Check sheet for the modelled part. Datum: model origin and axes. Units: mm. A direction names the side the tool comes from. Give positions to 0.01 mm unless a question says otherwise; leave off trailing zeros. Use one line per item in the form item = value.
from build123d import *

# Parameters (mm, degrees)
ESQUISSE1_R                               = 30
BOSS_EXTRU_1_DEPTH                        = 5
ESQUISSE6_R                               = 35
ESQUISSE6_R_2                             = 30
BOSS_EXTRU_6_DEPTH                        = 10
ESQUISSE7_R                               = 32.5
ESQUISSE7_R_2                             = 30
BOSS_EXTRU_8_DEPTH                        = 30
CONG_2_R                                  = 10
BOSS_EXTRU_9_DEPTH                        = 20
BOSS_EXTRU_10_DEPTH                       = 12
CHANFREIN1_SIZE                           = 6
CONG_3_R                                  = 5
ENL_V_MAT_EXTRU_1_REACH                   = 93.085
ENL_V_MAT_EXTRU_1_END_RADIUS              = 32.5
ESQUISSE10_R                              = 4.5
ESQUISSE11_R                              = 4.5
ESQUISSE11_R_2                            = 2.6
BOSS_EXTRU_11_DEPTH                       = 3
R_P_TITION_CIRCULAIRE1_COUNT              = 4
CHANFREIN1_OF_R_P_TITION_CIRCULAIRE1_SIZE = 6


# Some blends are built 0.0001 mm under size
with BuildPart() as part:
    # Esquisse1 → Boss.-Extru.1 (new body)
    with BuildSketch(Plane.XY):
        with BuildLine():
            Line((-10.847469364, 35.896830061), (-80, 15))
            Line((-80, 15), (-80, -15))
            Line((-80, -15), (-10.847469364, -35.896830061))
            ThreePointArc((-10.847469364, -35.896830061), (37.5, 0), (-10.847469364, 35.896830061))
        make_face()
        Circle(ESQUISSE1_R, mode=Mode.SUBTRACT)
    extrude(amount=BOSS_EXTRU_1_DEPTH)

    # Esquisse6 → Boss.-Extru.6 (add)
    with BuildSketch(Plane.XY.offset(5)):
        Circle(ESQUISSE6_R)
        Circle(ESQUISSE6_R_2, mode=Mode.SUBTRACT)
    extrude(amount=BOSS_EXTRU_6_DEPTH)

    # Esquisse7 → Boss.-Extru.8 (add)
    with BuildSketch(Plane.XY.offset(15)):
        Circle(ESQUISSE7_R)
        Circle(ESQUISSE7_R_2, mode=Mode.SUBTRACT)
    extrude(amount=BOSS_EXTRU_8_DEPTH)

    # Congé2
    # the kernel refuses this fillet: 10 mm, written as the material it adds along each edge
    with BuildSketch(Plane(origin=(0, 0, 15), x_dir=(1, 0, 0), z_dir=(0, -1, 0))) as cong_2_piece_1:
        with BuildLine():
            CenterArc((42.5, 6.614378278), CONG_2_R, 180, 41.409622109)
            Line((32.5, 6.614378278), (32.3, 6.614378278))
            Line((32.3, 6.614378278), (32.3, 0))
            Line((32.3, 0), (32.5, -0.2))
            ThreePointArc((32.5, -0.2), (33.75, -0.2), (34.85, -0.132287566))
            Line((34.85, -0.132287566), (35, 0))
        make_face()
    revolve(axis=Axis((0, 0, 15), (0, 0, 1)))

    # Esquisse8 → Boss.-Extru.9 (add)
    with BuildSketch(Plane.XY.offset(5)):
        with BuildLine():
            Line((-80, 15), (-37.080992435, 15))
            ThreePointArc((-37.080992435, 15), (-40, 0), (-37.080992435, -15))
            Line((-37.080992435, -15), (-80, -15))
            Line((-80, -15), (-80, 15))
        make_face()
    extrude(amount=BOSS_EXTRU_9_DEPTH)

    # Esquisse9 → Boss.-Extru.10 (add)
    with BuildSketch(Plane.XY.offset(45)):
        Polygon((-29.606282822, -13.405894878), (-22.723365586, -23.235719409), (-16.170149231, -18.647107918), (-23.053066468, -8.817283387), align=None)
    boss_extru_10 = extrude(amount=-BOSS_EXTRU_10_DEPTH)

    # Chanfrein1
    # the kernel refuses this chamfer: 6 mm, written as the material it adds along each edge
    with BuildSketch(Plane(origin=(0, 0, 33), x_dir=(-0.2418024484236128, -0.9703254999928355, 0), z_dir=(0.9703254999928355, -0.2418024484236128, 0))) as chanfrein1_piece_1_section:
        Polygon((30, CHANFREIN1_SIZE), (30 - CHANFREIN1_SIZE, 0), (30, 0), align=None)
    chanfrein1_piece_1 = revolve(axis=Axis((0, 0, 33), (0, 0, -1)), revolution_arc=82.01410645, mode=Mode.PRIVATE)
    chanfrein1_piece_1 = split(chanfrein1_piece_1, bisect_by=Plane(origin=(-19.354245876, -20.876636392, 31.008979001), z_dir=(-0.573576436351043, 0.819152044288994, 0)), keep=Keep.TOP, mode=Mode.PRIVATE)
    chanfrein1_piece_1 = split(chanfrein1_piece_1, bisect_by=Plane(origin=(-26.237163113, -11.04681186, 31.008979001), z_dir=(0.5735764363510415, -0.8191520442889951, 0)), keep=Keep.TOP, mode=Mode.PRIVATE)
    chanfrein1_piece_1 = split(chanfrein1_piece_1, bisect_by=Plane(origin=(-19.611607849, -13.732195653, 31.008979001), z_dir=(-0.8191520442889946, -0.5735764363510422, 0)), keep=Keep.TOP, mode=Mode.PRIVATE)
    add(chanfrein1_piece_1)

    # Congé3
    cong_3_edges = [part.edges().sort_by_distance(p)[0] for p in [
        (37.5, 0, 0),
        (-45.423734682, 25.44841503, 0),
        (-45.423734682, -25.44841503, 0),
    ]]
    fillet(cong_3_edges, radius=CONG_3_R - 0.0001)  # a hair under: the kernel refuses the full size

    # Enlèv. mat.-Extru.1: up to this cylinder (the profile starts inside it)
    enl_v_mat_extru_1_end = Plane(origin=(0, 0, 39), z_dir=(0, 0, -1)) * Cylinder(ENL_V_MAT_EXTRU_1_END_RADIUS, 252.17, mode=Mode.PRIVATE)
    # Esquisse10 → Enlèv. mat.-Extru.1 (cut, up to the surface)
    with BuildSketch(Plane(origin=(-19.611607849, -13.732195653, 0), x_dir=(0, 0, -1), z_dir=(0.8191520442889946, 0.5735764363510424, 0)), mode=Mode.PRIVATE) as enl_v_mat_extru_1_sk1:
        with Locations(Location((-39, 0, 0), (0, 0, 90))):
            Circle(ESQUISSE10_R)
    enl_v_mat_extru_1_tool1 = extrude(enl_v_mat_extru_1_sk1.sketch, amount=-ENL_V_MAT_EXTRU_1_REACH, mode=Mode.PRIVATE) & enl_v_mat_extru_1_end
    enl_v_mat_extru_1 = enl_v_mat_extru_1_tool1.solids().sort_by_distance((-19.611608, -13.732196, 39))[0]
    add(enl_v_mat_extru_1, mode=Mode.SUBTRACT)

    # Esquisse11 → Boss.-Extru.11 (add)
    with BuildSketch(Plane(origin=(-19.611607849, -13.732195653, 0), x_dir=(0, 0, -1), z_dir=(0.8191520442889946, 0.5735764363510424, 0))):
        with Locations(Location((-39, 0, 0), (0, 0, 90))):
            Circle(ESQUISSE11_R)
        with Locations(Location((-39, 0, 0), (0, 0, 90))):
            Circle(ESQUISSE11_R_2, mode=Mode.SUBTRACT)
    boss_extru_11 = extrude(amount=-BOSS_EXTRU_11_DEPTH)

    # Répétition circulaire1: Boss.-Extru.10, Enlèv. mat.-Extru.1, Boss.-Extru.11 ×4 about axis
    r_p_tition_circulaire1_axis = Axis((0, 0, 0), (0, 0, 1))
    add([boss_extru_10.rotate(r_p_tition_circulaire1_axis, i * 360 / R_P_TITION_CIRCULAIRE1_COUNT) for i in range(1, R_P_TITION_CIRCULAIRE1_COUNT)])
    add([enl_v_mat_extru_1.rotate(r_p_tition_circulaire1_axis, i * 360 / R_P_TITION_CIRCULAIRE1_COUNT) for i in range(1, R_P_TITION_CIRCULAIRE1_COUNT)], mode=Mode.SUBTRACT)
    add([boss_extru_11.rotate(r_p_tition_circulaire1_axis, i * 360 / R_P_TITION_CIRCULAIRE1_COUNT) for i in range(1, R_P_TITION_CIRCULAIRE1_COUNT)])

    # Chanfrein1 of Répétition circulaire1
    # the kernel refuses this chamfer: 6 mm, written as the material it adds along each edge
    with BuildSketch(Plane(origin=(0, 0, 33), x_dir=(0.9703254999928355, -0.24180244842361298, 0), z_dir=(0.24180244842361298, 0.9703254999928355, 0))) as chanfrein1_of_r_p_tition_circulaire1_piece_1_section:
        Polygon((30, CHANFREIN1_OF_R_P_TITION_CIRCULAIRE1_SIZE), (30 - CHANFREIN1_OF_R_P_TITION_CIRCULAIRE1_SIZE, 0), (30, 0), align=None)
    chanfrein1_of_r_p_tition_circulaire1_piece_1 = revolve(axis=Axis((0, 0, 33), (0, 0, -1)), revolution_arc=82.01410645, mode=Mode.PRIVATE)
    chanfrein1_of_r_p_tition_circulaire1_piece_1 = split(chanfrein1_of_r_p_tition_circulaire1_piece_1, bisect_by=Plane(origin=(20.876636392, -19.354245876, 31.008979001), z_dir=(-0.8191520442889941, -0.5735764363510429, 0)), keep=Keep.TOP, mode=Mode.PRIVATE)
    chanfrein1_of_r_p_tition_circulaire1_piece_1 = split(chanfrein1_of_r_p_tition_circulaire1_piece_1, bisect_by=Plane(origin=(11.04681186, -26.237163113, 31.008979001), z_dir=(0.8191520442889952, 0.5735764363510414, 0)), keep=Keep.TOP, mode=Mode.PRIVATE)
    chanfrein1_of_r_p_tition_circulaire1_piece_1 = split(chanfrein1_of_r_p_tition_circulaire1_piece_1, bisect_by=Plane(origin=(13.732195653, -19.611607849, 31.008979001), z_dir=(0.573576436351042, -0.8191520442889947, 0)), keep=Keep.TOP, mode=Mode.PRIVATE)
    add(chanfrein1_of_r_p_tition_circulaire1_piece_1)
    with BuildSketch(Plane(origin=(0, 0, 33), x_dir=(0.24180244842361312, 0.9703254999928353, 0), z_dir=(-0.9703254999928353, 0.24180244842361312, 0))) as chanfrein1_of_r_p_tition_circulaire1_piece_2_section:
        Polygon((30, CHANFREIN1_OF_R_P_TITION_CIRCULAIRE1_SIZE), (30 - CHANFREIN1_OF_R_P_TITION_CIRCULAIRE1_SIZE, 0), (30, 0), align=None)
    chanfrein1_of_r_p_tition_circulaire1_piece_2 = revolve(axis=Axis((0, 0, 33), (0, 0, -1)), revolution_arc=82.01410645, mode=Mode.PRIVATE)
    chanfrein1_of_r_p_tition_circulaire1_piece_2 = split(chanfrein1_of_r_p_tition_circulaire1_piece_2, bisect_by=Plane(origin=(19.354245876, 20.876636392, 31.008979001), z_dir=(0.5735764363510429, -0.8191520442889941, 0)), keep=Keep.TOP, mode=Mode.PRIVATE)
    chanfrein1_of_r_p_tition_circulaire1_piece_2 = split(chanfrein1_of_r_p_tition_circulaire1_piece_2, bisect_by=Plane(origin=(26.237163113, 11.04681186, 31.008979001), z_dir=(-0.5735764363510414, 0.8191520442889952, 0)), keep=Keep.TOP, mode=Mode.PRIVATE)
    chanfrein1_of_r_p_tition_circulaire1_piece_2 = split(chanfrein1_of_r_p_tition_circulaire1_piece_2, bisect_by=Plane(origin=(19.611607849, 13.732195653, 31.008979001), z_dir=(0.8191520442889947, 0.573576436351042, 0)), keep=Keep.TOP, mode=Mode.PRIVATE)
    add(chanfrein1_of_r_p_tition_circulaire1_piece_2)
    with BuildSketch(Plane(origin=(0, 0, 33), x_dir=(-0.9703254999928356, 0.24180244842361232, 0), z_dir=(-0.24180244842361232, -0.9703254999928356, 0))) as chanfrein1_of_r_p_tition_circulaire1_piece_3_section:
        Polygon((30, CHANFREIN1_OF_R_P_TITION_CIRCULAIRE1_SIZE), (30 - CHANFREIN1_OF_R_P_TITION_CIRCULAIRE1_SIZE, 0), (30, 0), align=None)
    chanfrein1_of_r_p_tition_circulaire1_piece_3 = revolve(axis=Axis((0, 0, 33), (0, 0, -1)), revolution_arc=82.01410645, mode=Mode.PRIVATE)
    chanfrein1_of_r_p_tition_circulaire1_piece_3 = split(chanfrein1_of_r_p_tition_circulaire1_piece_3, bisect_by=Plane(origin=(-20.876636392, 19.354245876, 31.008979001), z_dir=(0.8191520442889941, 0.5735764363510428, 0)), keep=Keep.TOP, mode=Mode.PRIVATE)
    chanfrein1_of_r_p_tition_circulaire1_piece_3 = split(chanfrein1_of_r_p_tition_circulaire1_piece_3, bisect_by=Plane(origin=(-11.04681186, 26.237163113, 31.008979001), z_dir=(-0.8191520442889952, -0.5735764363510413, 0)), keep=Keep.TOP, mode=Mode.PRIVATE)
    chanfrein1_of_r_p_tition_circulaire1_piece_3 = split(chanfrein1_of_r_p_tition_circulaire1_piece_3, bisect_by=Plane(origin=(-13.732195653, 19.611607849, 31.008979001), z_dir=(-0.5735764363510419, 0.8191520442889947, 0)), keep=Keep.TOP, mode=Mode.PRIVATE)
    add(chanfrein1_of_r_p_tition_circulaire1_piece_3)


solid = part.part
1) Set-up check for faces 4 (the face through (15.54, -22.03, 30.04)), 5 (the face through (-40, 0, 15)), 6 (the face through (-23.75, -13.05, 39.06)), 7 (the face through (-59, 15, 15)): record each of +Z, -Z, +X, -X, +Y, -Y from which the full face is reachable in a straight line by a thin tool's end or side.
Evaluation:
face_4 = -Z
face_5 = +Z
face_6 = none
face_7 = +Z, -X, +Y
2) Depth check by flat-ended pin: pin 1 Ø1.5 at (x, y) = (-13.5, 19.5) entering from -Z; pin 2 Ø6 at (x, z) = (-64, 15.5) entering from +Y; pin 3 Ø6 at (x, y) = (21.5, 6.5) entering from -Z. Enter the tip coordinate at first touch or a pass-through.
Evaluation:
pin_1 = 32.53
pin_2 = 15
pin_3 = 32.1
3) Scan lines: line 1 (Y direction, x = 0, z = 12); line 2 (X direction, y = -1, z = 41); line 3 (Y direction, x = 0, z = 32.5). Record each from-to range of solid material in increasing order.
Evaluation:
line_1 = -35 to -30, 30 to 35
line_2 = -32.48 to -29.98, 29.98 to 32.48
line_3 = -32.5 to -30, 30 to 32.5
4) Release check for a two-part mould opening along Z. For faces 1 (the face through (15.04, -20.5, 36.46)), 2 (the face through (-80, 0, 12)), 3 (the face through (22.03, 15.54, 30.04)) record: pulls with the +Z half, pulls with the -Z half, needs draft (parallel to the pull), parting line crosses it, or undercut.
Evaluation:
face_1 = undercut
face_2 = needs draft
face_3 = pulls with the -Z half
